Here's how the part is built. I have some questions about the finished solid (model axes, mm). A direction names the side the tool comes from. Give positions to 0.01 mm unless a question says otherwise; leave off trailing zeros. Write each loop counter-clockwise with the first axis right and the second up, starting at its lowest first coordinate (ties: lowest second). Pieces come first, ordered by that corner, then holes. Notation, with made-up numbers: (6, 79.25) -> (49, 79.25) arc R27 ccw to (49, 97.25) -> close; hole circle Ø4 at (-6, 75.5). An arc over 180 degrees is marked (long way). Put each result on its own line as item: value. Start each with the question number.
from build123d import *

# Parameters (mm, degrees)
SKETCH1_W           = 195.2625
SKETCH1_H           = 40.64
SKETCH1_R           = 2.4892
BOSS_EXTRUDE1_DEPTH = 17.78
SKETCH2_R           = 3.96875
CUT_EXTRUDE1_DEPTH  = 40.64
SKETCH3_R           = 4.064
CUT_EXTRUDE2_DEPTH  = 4.7752
CUT_EXTRUDE3_DEPTH  = 17.78
FILLET1_R           = 2.54


with BuildPart() as part:
    # Sketch1 → Boss-Extrude1 (new body)
    with BuildSketch(Plane.XY):
        with Locations((-88.9, 0)):
            Rectangle(SKETCH1_W, SKETCH1_H)
        Circle(SKETCH1_R, mode=Mode.SUBTRACT)
        with Locations((-177.8, 0)):
            Circle(SKETCH1_R, mode=Mode.SUBTRACT)
        with Locations((-88.9, 0)):
            Circle(SKETCH1_R, mode=Mode.SUBTRACT)
    extrude(amount=-BOSS_EXTRUDE1_DEPTH)

    # Sketch2 → Cut-Extrude1 (cut)
    with BuildSketch(Plane(origin=(0, 20.32, 0), x_dir=(1, 0, 0), z_dir=(0, 1, 0))):
        with Locations(Location((-12.7, 8.89, 0), (0, 0, 270))):
            Circle(SKETCH2_R)
        with Locations(Location((-63.5, 8.89, 0), (0, 0, 270))):
            Circle(SKETCH2_R)
        with Locations(Location((-114.3, 8.89, 0), (0, 0, 270))):
            Circle(SKETCH2_R)
        with Locations(Location((-165.1, 8.89, 0), (0, 0, 270))):
            Circle(SKETCH2_R)
    extrude(amount=-CUT_EXTRUDE1_DEPTH, mode=Mode.SUBTRACT)

    # Sketch3 → Cut-Extrude2 (cut)
    with BuildSketch(Plane.XY):
        Circle(SKETCH3_R)
        with Locations((-88.9, 0)):
            Circle(SKETCH3_R)
        with Locations((-177.8, 0)):
            Circle(SKETCH3_R)
    extrude(amount=-CUT_EXTRUDE2_DEPTH, mode=Mode.SUBTRACT)

    # Sketch5 → Cut-Extrude3 (cut)
    with BuildSketch(Plane.XY):
        with BuildLine():
            Line((0, -20.32), (8.73125, -20.32))
            Line((8.73125, -20.32), (8.73125, 20.32))
            Line((8.73125, 20.32), (0, 20.32))
            Line((0, 20.32), (0, 10.622546022))
            ThreePointArc((0, 10.622546022), (0.546012526, 9.049137635), (1.949302326, 8.152186482))
            ThreePointArc((1.949302326, 8.152186482), (8.382, 0), (1.949302326, -8.152186482))
            ThreePointArc((1.949302326, -8.152186482), (0.546012526, -9.049137635), (0, -10.622546022))
            Line((0, -10.622546022), (0, -20.32))
        make_face()
        with BuildLine():
            Line((-22.86, -15.24), (-53.34, -15.24))
            ThreePointArc((-53.34, -15.24), (-55.136051224, -14.496051224), (-55.88, -12.7))
            Line((-55.88, -12.7), (-55.88, 12.7))
            ThreePointArc((-55.88, 12.7), (-55.136051224, 14.496051224), (-53.34, 15.24))
            Line((-53.34, 15.24), (-22.86, 15.24))
            ThreePointArc((-22.86, 15.24), (-21.063948776, 14.496051224), (-20.32, 12.7))
            Line((-20.32, 12.7), (-20.32, -12.7))
            ThreePointArc((-20.32, -12.7), (-21.063948776, -14.496051224), (-22.86, -15.24))
        make_face()
        with BuildLine():
            Line((-85.011936327, -9.38661605), (-85.011936327, -13.97))
            ThreePointArc((-85.011936327, -13.97), (-84.639961939, -14.868025612), (-83.741936327, -15.24))
            Line((-83.741936327, -15.24), (-73.66, -15.24))
            ThreePointArc((-73.66, -15.24), (-71.863948776, -14.496051224), (-71.12, -12.7))
            Line((-71.12, -12.7), (-71.12, 12.7))
            ThreePointArc((-71.12, 12.7), (-71.863948776, 14.496051224), (-73.66, 15.24))
            Line((-73.66, 15.24), (-83.741936327, 15.24))
            ThreePointArc((-83.741936327, 15.24), (-84.639961939, 14.868025612), (-85.011936327, 13.97))
            Line((-85.011936327, 13.97), (-85.011936327, 9.38661605))
            ThreePointArc((-85.011936327, 9.38661605), (-78.74, 0), (-85.011936327, -9.38661605))
        make_face()
        with BuildLine():
            Line((-104.14, 15.24), (-94.058063673, 15.24))
            ThreePointArc((-94.058063673, 15.24), (-93.160038061, 14.868025612), (-92.788063673, 13.97))
            Line((-92.788063673, 13.97), (-92.788063673, 9.38661605))
            ThreePointArc((-92.788063673, 9.38661605), (-99.06, 0), (-92.788063673, -9.38661605))
            Line((-92.788063673, -9.38661605), (-92.788063673, -13.97))
            ThreePointArc((-92.788063673, -13.97), (-93.160038061, -14.868025612), (-94.058063673, -15.24))
            Line((-94.058063673, -15.24), (-104.14, -15.24))
            ThreePointArc((-104.14, -15.24), (-105.936051224, -14.496051224), (-106.68, -12.7))
            Line((-106.68, -12.7), (-106.68, 12.7))
            ThreePointArc((-106.68, 12.7), (-105.936051224, 14.496051224), (-104.14, 15.24))
        make_face()
        with BuildLine():
            Line((-154.94, 15.24), (-124.46, 15.24))
            ThreePointArc((-124.46, 15.24), (-122.663948776, 14.496051224), (-121.92, 12.7))
            Line((-121.92, 12.7), (-121.92, -12.7))
            ThreePointArc((-121.92, -12.7), (-122.663948776, -14.496051224), (-124.46, -15.24))
            Line((-124.46, -15.24), (-154.94, -15.24))
            ThreePointArc((-154.94, -15.24), (-156.736051224, -14.496051224), (-157.48, -12.7))
            Line((-157.48, -12.7), (-157.48, 12.7))
            ThreePointArc((-157.48, 12.7), (-156.736051224, 14.496051224), (-154.94, 15.24))
        make_face()
        with BuildLine():
            Line((-186.53125, -20.32), (-186.53125, 20.32))
            Line((-186.53125, 20.32), (-177.8, 20.32))
            Line((-177.8, 20.32), (-177.8, 10.622546022))
            ThreePointArc((-177.8, 10.622546022), (-178.346012526, 9.049137635), (-179.749302326, 8.152186482))
            ThreePointArc((-179.749302326, 8.152186482), (-186.182, 0), (-179.749302326, -8.152186482))
            ThreePointArc((-179.749302326, -8.152186482), (-178.346012526, -9.049137635), (-177.8, -10.622546022))
            Line((-177.8, -10.622546022), (-177.8, -20.32))
            Line((-177.8, -20.32), (-186.53125, -20.32))
        make_face()
    extrude(amount=-CUT_EXTRUDE3_DEPTH, mode=Mode.SUBTRACT)

    # Fillet1
    fillet1_edges = [part.edges().sort_by_distance(p)[0] for p in [
        (0, 20.32, -8.89),
        (0, -20.32, -8.89),
        (-177.8, -20.32, -8.89),
        (-177.8, 20.32, -8.89),
    ]]
    fillet(fillet1_edges, radius=FILLET1_R)


solid = part.part
1) I'm going to push flat-ended pins straight in: pin 1 Ø5.5 at (y, z) = (6, -10.5) entering from -X; pin 2 Ø3 at (y, z) = (-13.5, -3.5) entering from -X; pin 3 Ø6.5 at (x, z) = (-12.7, -8.89) entering from -Y; pin 4 Ø3.5 at (y, z) = (13, -5) entering from +X. Where does each tip first touch, or does it pass through?
2) Which directions (+Z, -Z, +X, -X, +Y, -Y) give clear straight access to the entire face, cutting with the end or side of a thin tool? Please do faces 5 (the flat face through (-177.8, -14, -9)), 6 (the flat face through (-38, 15.24, -9)), 7 (the flat face through (0, 14, -9)).
3) I want a section at A-A, the plane x = -12.7. Write out the boundary of the cut face in (y, z), and give its area (3 significant figures).
4) I want a section at B-B, the plane z = -8.89. State how many separate pieces and enclosed holes the cut face has, and give its area (3 significant figures).
5) I need wall thicknesses on probe 1 along X at (y, z) = (-15, -1.25); probe 2 along Y at (x, z) = (-80, -9.5); probe 3 along X at (y, z) = (9, -13.25). Which ranges of each line are inside material? Lowest first, please.
6) I want a section at C-C, the plane x = -51.5. Write out the boundary of the cut face in (y, z), and give its area (3 significant figures).
7) Thinking about a two-plate mould opening in Y: for faces 1 (the flat face through (-90, -20.32, -9)), 2 (the flat face through (-90, 20.32, -9)), 3 (the flat face through (-90, 5, 0)), 4 (the flat face through (-106.68, 0, -9)), which applies, released by +Y, released by -Y, zero draft, split by the parting line, or undercut?
Established:
1. pin 1: stops at x = -185.53
1. pin 2: stops at x = -177.8
1. pin 3: passes through
1. pin 4: stops at x = 0
2. face 5: +Z, -Z, -X, -Y
2. face 6: +Z, -Z
2. face 7: +Z, -Z, +X, +Y
3. outline: (-20.32, -17.78) -> (20.32, -17.78) -> (20.32, -12.86) -> (-20.32, -12.86) -> close; (-20.32, -4.92) -> (20.32, -4.92) -> (20.32, 0) -> (-20.32, 0) -> close
3. area: 400 mm2
4. separate pieces: 5
4. enclosed holes: 7
4. area: 3,270 mm2
5. probe 1: x = -177.8 to -156.02, -123.38 to -105.22, -93.32 to -84.48, -72.58 to -54.42, -21.78 to 0
5. probe 2: y = -20.32 to -15.24, -4.9 to 4.9, 15.24 to 20.32
5. probe 3: x = -178.39 to -157.48, -121.92 to -106.68, -93.61 to -84.19, -71.12 to -55.88, -20.32 to 0.59
6. outline: (-20.32, -17.78) -> (-15.24, -17.78) -> (-15.24, 0) -> (-20.32, 0) -> close; (15.24, -17.78) -> (20.32, -17.78) -> (20.32, 0) -> (15.24, 0) -> close
6. area: 181 mm2
7. face 1: released by -Y
7. face 2: released by +Y
7. face 3: zero draft
7. face 4: undercut
